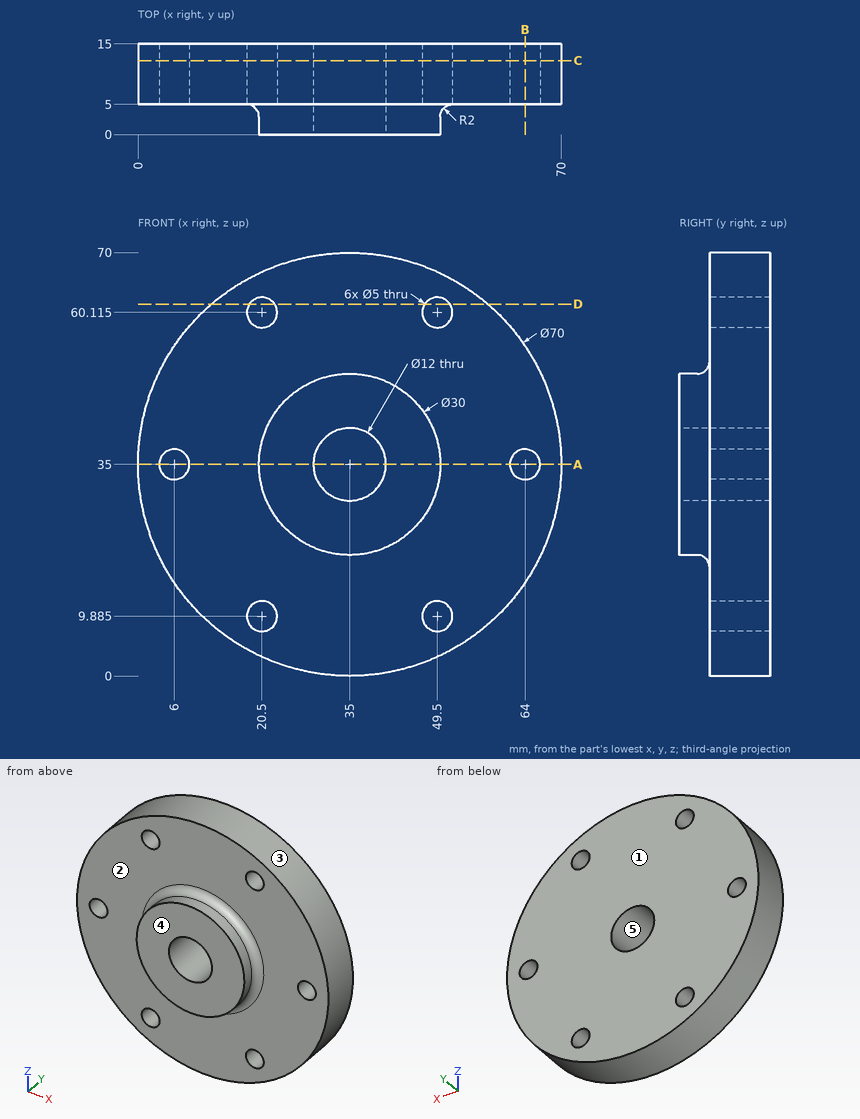
Geometry: see drawing. Coordinates: mm, zero at the bounding-box minimum. A direction names the side the tool comes from. Give positions to 0.01 mm unless a question says otherwise; leave off trailing zeros. Order: outer loops, then holes, each group sorted by start corner. A loop starts at its lowest first (then second) coordinate and runs counter-clockwise, first axis right, second up. Notation, with made-up numbers: (45.5, -26) - (91.5, -26) arc R27 ccw to (91.5, -3) - close; hole circle Ø10 at (76, -35.5). An arc over 180 degrees is marked (long way). Use CSV: the item, a comma, the result in double quotes.
1. Material intervals for line 1 along X through (y, z) = (8, 34.5); line 2 along Y through (x, z) = (29.5, 64); line 3 along X through (y, z) = (9, 9), sorted ascending. Write a range as from..to.
Answers below:
line 1,"0..3.55, 8.45..29.02, 40.98..61.55, 66.45..70"
line 2,"5..15"
line 3,"11.57..18.16, 22.84..47.16, 51.84..58.43"
2. Access query for the marked faces 1 and 2. Directions: +Z, -Z, +X, -X, +Y, -Y. A direction counts if a zero-diameter tool reaches every point of the face in a straight line with its end or side. Return the directions, or none.
Answers below:
face 1,"+Z, -Z, +X, -X, +Y"
face 2,"-Y"
3. Section query A-A (z = 35). Output: boundary loops of the cut face in (x, y).
Answers below:
outline,"(0, 5) - (3.5, 5) - (3.5, 15) - (0, 15) - close; (8.5, 5) - (18, 5) arc R2 cw to (20, 3) - (20, 0) - (29, 0) - (29, 15) - (8.5, 15) - close; (41, 0) - (50, 0) - (50, 3) arc R2 cw to (52, 5) - (61.5, 5) - (61.5, 15) - (41, 15) - close; (66.5, 5) - (70, 5) - (70, 15) - (66.5, 15) - close"
4. Mould query, pull axis Z, two halves, no side actions, for the marked faces 3, 4 and 5. Classes: +Z half, -Z half, draft (parallel to the pull), parting line (faces both ways), or undercut.
Answers below:
face 3,"parting line"
face 4,"draft"
face 5,"undercut"
5. Section query C-C (y = 12.25). Give the number of separate pieces and of enclosed holes in the cut face, plus the area to 3 significant figures.
Answers below:
separate pieces,"1"
enclosed holes,"7"
area,"3,620 mm2"
6. Section query B-B (x = 64). Output: boundary loops of the cut face in (y, z).
Answers below:
outline,"(5, 15.4) - (15, 15.4) - (15, 32.5) - (5, 32.5) - close; (5, 37.5) - (15, 37.5) - (15, 54.6) - (5, 54.6) - close"
7. Contact query for flat-ended pins moving along their axis: pin 1 (5 mm diameter, centred on y = 4.5, z = 15, fed in from +X); pin 2 (2 mm diameter, centred on x = 45, y = 7.5, fed in from -Z); pin 3 (6 mm diameter, centred on y = 3.5, z = 10, fed in from +X); pin 4 (4 mm diameter, centred on x = 6, z = 35, fed in from -Y). Output: stop coordinate, or through.
Answers below:
pin 1,"x = 65.28"
pin 2,"z = 1.18"
pin 3,"x = 61.89"
pin 4,"through"
8. Section query D-D (z = 61.5). Output: boundary loops of the cut face in (x, y), plus the area to 3 significant figures.
Answers below:
outline,"(12.14, 5) - (18.42, 5) - (18.42, 15) - (12.14, 15) - close; (22.58, 5) - (47.42, 5) - (47.42, 15) - (22.58, 15) - close; (51.58, 5) - (57.86, 5) - (57.86, 15) - (51.58, 15) - close"
area,"374 mm2"
